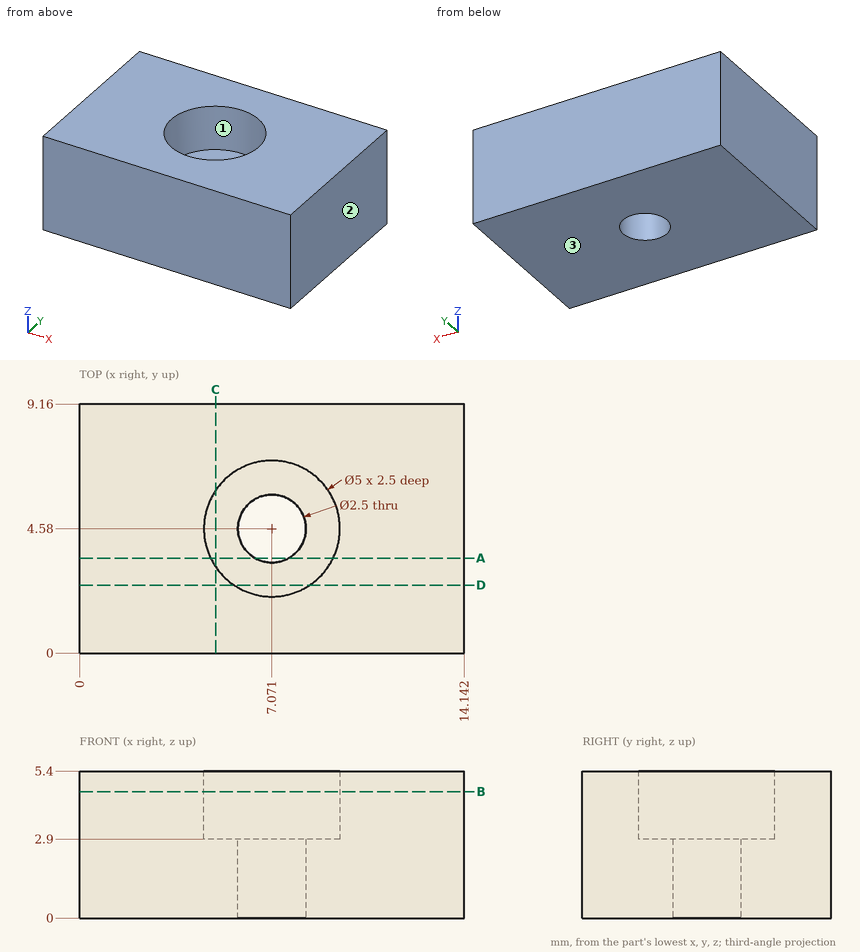
Geometry check sheet. Reference: drawing and pictorial views, mm from the part's lowest x, y, z. Round coordinates to 2 decimals unless told otherwise and drop trailing zeros. Order: outer loops, then holes, each group sorted by start corner. A loop starts at its lowest first (then second) coordinate and runs counter-clockwise, first axis right, second up. Notation, with made-up numbers: (38, 85) - (52, 85) arc R21 ccw to (52, 98) - close; hole circle Ø6 at (16.25, 57.5). An arc over 180 degrees is marked (long way). Use a Markdown table: item, result. Add a question column.
1) Section check B-B (z = 4.65). Record the cut outline in (x, y).
2) Thickness scan on line 1 along Y through (x, z) = (9, 3.1); line 2 along X through (y, z) = (3.5, 0.35); line 3 along X through (y, z) = (5.25, 2.6) (1 decimal). Record the ranges inside material, lowest first.
3) Section check A-A (y = 3.5). Record the cut outline in (x, z).
4) Section check D-D (y = 2.5). Record the cut outline in (x, z).
5) Mould release check, pull along X, two halves, no side actions. Record for the marked faces 1, 2 and 3: released by +X, released by -X, zero draft, split by the parting line, or undercut.
6) Section check C-C (x = 5). Record the cut outline in (y, z).
7) Gauge pin test, flat end, axial feed: P1, Ø4, axis at x = 7.07, y = 4.58, coming from the +Z side. Record the tip position at first contact, or that the pin passes through.
Established:
| question | item | result |
|---|---|---|
| 1 | outline | (0, 0) - (14.14, 0) - (14.14, 9.16) - (0, 9.16) - close; hole circle Ø5 at (7.07, 4.58) |
| 2 | line 1 | 0 to 2.99, 6.17 to 9.16 |
| 2 | line 2 | 0 to 6.44, 7.7 to 14.14 |
| 2 | line 3 | 0 to 6, 8.1 to 14.1 |
| 3 | outline | (0, 0) - (6.44, 0) - (6.44, 2.9) - (4.82, 2.9) - (4.82, 5.4) - (0, 5.4) - close; (7.7, 0) - (14.14, 0) - (14.14, 5.4) - (9.33, 5.4) - (9.33, 2.9) - (7.7, 2.9) - close |
| 4 | outline | (0, 0) - (14.14, 0) - (14.14, 5.4) - (8.46, 5.4) - (8.46, 2.9) - (5.68, 2.9) - (5.68, 5.4) - (0, 5.4) - close |
| 5 | face 1 | undercut |
| 5 | face 2 | released by +X |
| 5 | face 3 | zero draft |
| 6 | outline | (0, 0) - (9.16, 0) - (9.16, 5.4) - (5.98, 5.4) - (5.98, 2.9) - (3.18, 2.9) - (3.18, 5.4) - (0, 5.4) - close |
| 7 | P1 | z = 2.9 |
